Could you check a few things on this model? Use its own coordinates, in mm. Face numbers are marked on the shaded views. A direction names the side the tool comes from. Coordinates: 2 decimals unless noted, no trailing zeros. Loops run counter-clockwise (first coordinate to the right, second up) from the corner with the lowest first, then second, coordinate; pieces in that order, holes last.
1) Imagine slicing it at D-D on z = 4. Please give me the cut outline in (x, y), plus the area to 3 significant figures.
2) Imagine slicing it at C-C on x = 9. Please give me the cut outline in (y, z).
3) If I drill on line 1 along Y through (x, z) = (0, -0.9); line 2 along Z through (x, y) = (4.5, -4.75); line 3 along X through (y, z) = (0.5, 6.5), over which ranges is the centre line in solid material (lowest first)?
4) Thinking about a two-plate mould opening in X: for the marked faces 3 and 4, which applies, released by +X, released by -X, zero draft, split by the parting line, or undercut?
5) Will these pins go through, and if not, where does the flat tip stop? P1, Ø5, axis at y = 5, z = 1.5, coming from the -X side; P2, Ø1, axis at y = 3.5, z = 1, coming from the +X side.
6) Imagine slicing it at B-B on y = -0.5. Please give me the cut outline in (x, z).
7) Imagine slicing it at A-A on x = 0. Please give me the cut outline in (y, z).
8) For the marked faces 1 and 2, which set-ups out of +Z, -Z, +X, -X, +Y, -Y let a thin tool reach every point of the face, with its end or its side?
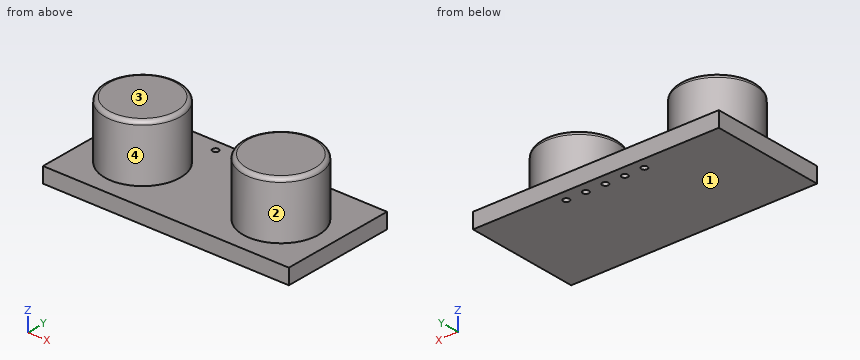
Autodesk Inventor part; units mm, degrees
ref_plane "YZ Plane" through (0, 0, 0) normal (1, 0, 0) x (0, 1, 0)
ref_plane "XZ Plane" through (0, 0, 0) normal (0, 1, 0) x (-1, 0, 0)
ref_plane "XY Plane" through (0, 0, 0) normal (0, 0, 1) x (1, 0, 0)
sketch "Sketch1" plane through (0, 0, 0) normal (0, 0, 1) x (1, 0, 0)
  line L0 (-16, 7.5) -> (16, 7.5)
  line L1 (16, 7.5) -> (16, -7.5)
  line L2 (16, -7.5) -> (-16, -7.5)
  line L3 (-16, -7.5) -> (-16, 7.5)
  line L4 (-16, 0) -> (-16, 7.5)
  line L5 (-16, 7.5) -> (0, 7.5)
  point P0 (0, 0)
  dimension "d0" = 32
  dimension "d1" = 15
extrude "Extrusion1" add sketch "Sketch1" against normal blind 2
sketch "Sketch2" plane through (0, 0, 0) normal (0, 0, 1) x (1, 0, 0)
  line L0 (-16, 7.5) -> (16, 7.5)
  line L1 (-16, -7.5) -> (-16, 7.5)
  line L2 (16, -7.5) -> (-16, -7.5)
  line L3 (16, 7.5) -> (16, -7.5)
  circle A0 centre (-9, -0.5) radius 4.9
  circle A1 centre (9, -0.5) radius 4.9
  circle A2 centre (0, 6.06) radius 0.4
  circle A3 centre (-2.54, 6.06) radius 0.4
  circle A4 centre (-5.08, 6.06) radius 0.4
  line L4 (0, 0) -> (0, 3) construction
  line L5 (0, 3) -> (0, 0) construction
  line L6 (16, 7.5) -> (-16, 7.5)
  circle A5 centre (2.54, 6.06) radius 0.4
  circle A6 centre (5.08, 6.06) radius 0.4
  point P0 (8.9861, 0.5)
  dimension "d8" = 9.8
  dimension "d11" = 32
  dimension "d12" = 15
  dimension "d16" = 8
  dimension "d17" = 9.8
  dimension "d19" = 9
  dimension "d20" = 9
  dimension "d24" = 0.8
  dimension "d25" = 1.44
  dimension "d26" = 0.8
  dimension "d27" = 2.54
  dimension "d28" = 0.8
  dimension "d29" = 2.54
extrude "Extrusion3" add sketch "Sketch2" along normal blind 7.4 contours A0 | A1
fillet "Fillet2" radius 0.5 2 edges at (-13.9, -0.5, 7.4) (4.1, -0.5, 7.4)
extrude "Extrusion4" cut sketch "Sketch2" against normal up to next contours A2 | A3 | A4 | A5 | A6
properties part number "srf10"
Filled in:
1. outline: circle Ø9.8 at (-9, -0.5); circle Ø9.8 at (9, -0.5)
1. area: 151 mm2
2. outline: (-7.5, -2) - (7.5, -2) - (7.5, 0) - (4.4, 0) - (4.4, 6.9) arc R0.5 ccw to (3.9, 7.4) - (-4.9, 7.4) arc R0.5 ccw to (-5.4, 6.9) - (-5.4, 0) - (-7.5, 0) - close
3. line 1: y = -7.5 to 5.66, 6.46 to 7.5
3. line 2: z = -2 to 0
3. line 3: x = -13.8 to -4.2, 4.2 to 13.8
4. face 3: zero draft
4. face 4: undercut
5. P1: stops at x = -16
5. P2: stops at x = 12.43
6. outline: (-16, -2) - (16, -2) - (16, 0) - (13.9, 0) - (13.9, 6.9) arc R0.5 ccw to (13.4, 7.4) - (4.6, 7.4) arc R0.5 ccw to (4.1, 6.9) - (4.1, 0) - (-4.1, 0) - (-4.1, 6.9) arc R0.5 ccw to (-4.6, 7.4) - (-13.4, 7.4) arc R0.5 ccw to (-13.9, 6.9) - (-13.9, 0) - (-16, 0) - close
7. outline: (-7.5, -2) - (5.66, -2) - (5.66, 0) - (-7.5, 0) - close; (6.46, -2) - (7.5, -2) - (7.5, 0) - (6.46, 0) - close
8. face 1: -Z, +X, -X, +Y, -Y
8. face 2: +Z
